The model under review builds one solid part; all positions refer to its coordinate system, in mm. Face numbers are marked on the shaded views. Round coordinates to 2 decimals unless told otherwise and drop trailing zeros. Loops run counter-clockwise (first coordinate to the right, second up) from the corner with the lowest first, then second, coordinate; pieces in that order, holes last. Notation, with made-up numbers: M 77.25,75 L 98.25,75 A27 cw 98.25,92 Z; hole C 33,-31 d1. An arc over 180 degrees is marked long. Answer as a JSON object with one key per item and string values. Group by question number.
Item 1: Consider section B-B (y = 23.5). Give the boundary of the cut face in (x, z) (3 decimals).
Item 2: Consider section C-C (x = -3). Give the boundary of the cut face in (y, z) (3 decimals).
Item 3: The part is to be moulded in two halves that separate along Z. For the marked faces 1 and 2, say which applies: +Z half, -Z half, draft (parallel to the pull), parting line (faces both ways), or undercut.
Item 4: To check wall thickness, follow line 1 (Y direction, x = 30, z = 2.2); line 2 (X direction, y = 0, z = 1.2); line 3 (X direction, y = 1.5, z = 2.95). State the ranges of each line that lie inside material, in increasing order.
Item 5: Consider section A-A (x = 30). Give the boundary of the cut face in (y, z) (3 decimals), and give its area (3 significant figures).
Item 6: Consider section D-D (y = 1.5). Give the boundary of the cut face in (x, z) (3 decimals), and give its area (3 significant figures).
Item 7: Insertion check: P1, Ø2.5, axis at x = -30, y = -23.5, coming from the +Z side; P2, Ø3, axis at x = 5.5, y = 16, coming from the -Z side; P3, Ø1.6, axis at y = 30.5, z = 1, coming from the -X side; P4, Ø1, axis at y = 29.5, z = 2.5, coming from the +X side. Each pin has a flat end and moves straight along its axis. Give the tip position at first contact, or say it passes through.
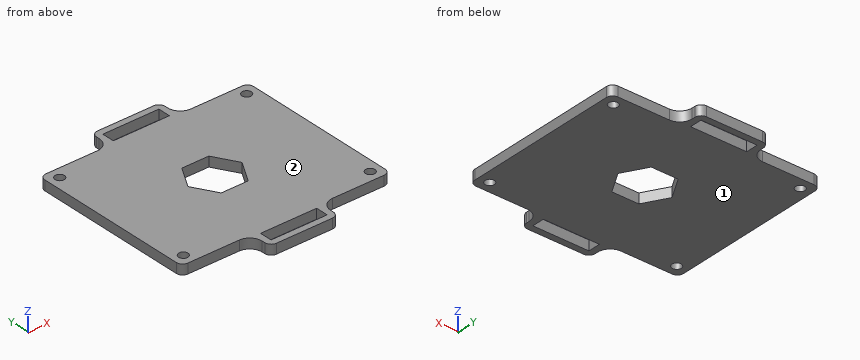
```python
from build123d import *

# Parameters (mm, degrees)
SKETCH1_R           = 1.5
SKETCH1_W           = 18
SKETCH1_H           = 4
BOSS_EXTRUDE1_DEPTH = 3.175
FILLET1_R           = 4
FILLET2_R           = 2


with BuildPart() as part:
    # Sketch1 → Boss-Extrude1 (new body)
    with BuildSketch(Plane.XY):
        Polygon((-33.5, 27), (-11, 27), (-11, 34), (11, 34), (11, 27), (33.5, 27), (33.5, -27), (11, -27), (11, -34), (-11, -34), (-11, -27), (-33.5, -27), align=None)
        with Locations((-30, 23.5)):
            Circle(SKETCH1_R, mode=Mode.SUBTRACT)
        with Locations((30, 23.5)):
            Circle(SKETCH1_R, mode=Mode.SUBTRACT)
        with Locations((30, -23.5)):
            Circle(SKETCH1_R, mode=Mode.SUBTRACT)
        with Locations((-30, -23.5)):
            Circle(SKETCH1_R, mode=Mode.SUBTRACT)
        with Locations((0, -30)):
            Rectangle(SKETCH1_W, SKETCH1_H, mode=Mode.SUBTRACT)
        with Locations((0, 30)):
            Rectangle(SKETCH1_W, SKETCH1_H, mode=Mode.SUBTRACT)
        Polygon((8.660254038, 0), (4.330127019, 7.5), (-4.330127019, 7.5), (-8.660254038, 0), (-4.330127019, -7.5), (4.330127019, -7.5), align=None, mode=Mode.SUBTRACT)
    extrude(amount=BOSS_EXTRUDE1_DEPTH)

    # Fillet1
    fillet1_edges = [part.edges().sort_by_distance(p)[0] for p in [
        (-11, 27, 1.5875),
        (11, 27, 1.5875),
        (11, -27, 1.5875),
        (-11, -27, 1.5875),
    ]]
    fillet(fillet1_edges, radius=FILLET1_R)

    # Fillet2
    fillet2_edges = [part.edges().sort_by_distance(p)[0] for p in [
        (-33.5, 27, 1.5875),
        (-11, 34, 1.5875),
        (11, 34, 1.5875),
        (33.5, 27, 1.5875),
        (33.5, -27, 1.5875),
        (11, -34, 1.5875),
        (-11, -34, 1.5875),
        (-33.5, -27, 1.5875),
    ]]
    fillet(fillet2_edges, radius=FILLET2_R)


solid = part.part
```
Geometry results:
{
 "1": {"outline": "M -33.5,0 L -31.5,0 L -31.5,3.175 L -33.5,3.175 Z; M -28.5,0 L 28.5,0 L 28.5,3.175 L -28.5,3.175 Z; M 31.5,0 L 33.5,0 L 33.5,3.175 L 31.5,3.175 Z"},
 "2": {"outline": "M -34,0 L -32,0 L -32,3.175 L -34,3.175 Z; M -28,0 L -7.5,0 L -7.5,3.175 L -28,3.175 Z; M 7.5,0 L 28,0 L 28,3.175 L 7.5,3.175 Z; M 32,0 L 34,0 L 34,3.175 L 32,3.175 Z"},
 "3": {"face 1": "-Z half", "face 2": "+Z half"},
 "4": {"line 1": "y = -27 to -25, -22 to 22, 25 to 27", "line 2": "x = -33.5 to -8.66, 8.66 to 33.5", "line 3": "x = -33.5 to -7.79, 7.79 to 33.5"},
 "5": {"outline": "M -27,0 L -25,0 L -25,3.175 L -27,3.175 Z; M -22,0 L 22,0 L 22,3.175 L -22,3.175 Z; M 25,0 L 27,0 L 27,3.175 L 25,3.175 Z", "area": "152 mm^2"},
 "6": {"outline": "M -33.5,0 L -7.794,0 L -7.794,3.175 L -33.5,3.175 Z; M 7.794,0 L 33.5,0 L 33.5,3.175 L 7.794,3.175 Z", "area": "163 mm^2"},
 "7": {"P1": "passes through", "P2": "stops at z = 0", "P3": "stops at x = -11.22", "P4": "stops at x = 11.54"}
}
